Verification items for the finished model (mm, model axes). Round coordinates to 2 decimals unless told otherwise and drop trailing zeros. Write each loop counter-clockwise with the first axis right and the second up, starting at its lowest first coordinate (ties: lowest second). Pieces come first, ordered by that corner, then holes.
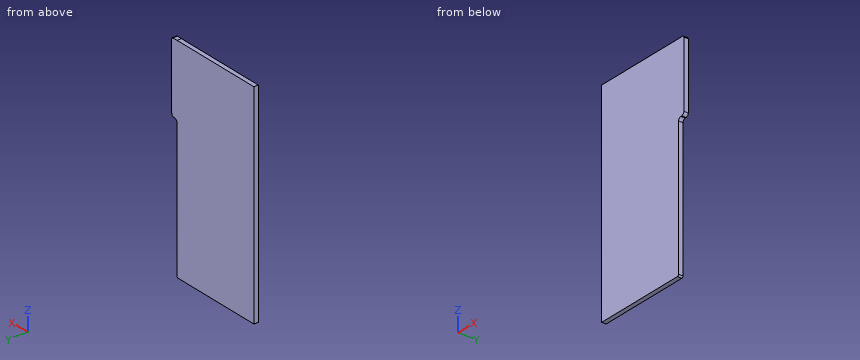
from build123d import *

# Parameters (mm, degrees)
F0_W     = 207.9625
F0_H     = 460.375
F1_DEPTH = 9.525
F2_W     = 14.2875
F2_H     = 153.458333
F3_DEPTH = 9.525
F4_R     = 3.175
F5_R     = 6.35


with BuildPart() as f1:
    # F0 (on Front) → F1 (new body)
    with BuildSketch(Plane.XZ):
        Rectangle(F0_W, F0_H)
    extrude(amount=F1_DEPTH)

    # F2 (on Front) → F3 (join, through all)
    with BuildSketch(Plane.XZ):
        with Locations((111.125, 153.458333)):
            Rectangle(F2_W, F2_H)
    extrude(amount=F3_DEPTH)

    # F4
    f4_edges = [f1.edges().sort_by_distance(p)[0] for p in [
        (103.98125, -4.7625, -230.1875),
        (118.26875, -4.7625, 230.1875),
    ]]
    fillet(f4_edges, radius=F4_R)

    # F5
    f5_edges = [f1.edges().sort_by_distance(p)[0] for p in [
        (103.98125, -4.7625, 76.729167),
        (118.26875, -4.7625, 76.729167),
    ]]
    fillet(f5_edges, radius=F5_R)


solid = f1.part
Q1. Material ranges on line 1 along X through (y, z) = (-5.5, -32.5); line 2 along X through (y, z) = (-5.75, 79.5); line 3 along Z through (x, y) = (104.5, -7.5), recorded low to high.
Recorded:
line 1: x = -103.98 to 103.98
line 2: x = -103.98 to 117.16
line 3: z = 72.89 to 230.19
Q2. Sectioned sample at B-B (z = -142.5). Enter the section's corners in (x, y) (3 decimals), plus the area to 3 significant figures.
Recorded:
outline: (-103.981, -9.525) - (103.981, -9.525) - (103.981, 0) - (-103.981, 0) - close
area: 1,980 mm2
Q3. Depth check by flat-ended pin: P1, Ø1.7, axis at x = 111.5, y = -4, coming from the -Z side; P2, Ø3, axis at y = -4.5, z = -144, coming from the +X side; P3, Ø4, axis at x = -44, z = 119.5, coming from the +Y side. Enter the tip coordinate at first touch or a pass-through.
Recorded:
P1: stops at z = 76.73
P2: stops at x = 103.98
P3: stops at y = 0
